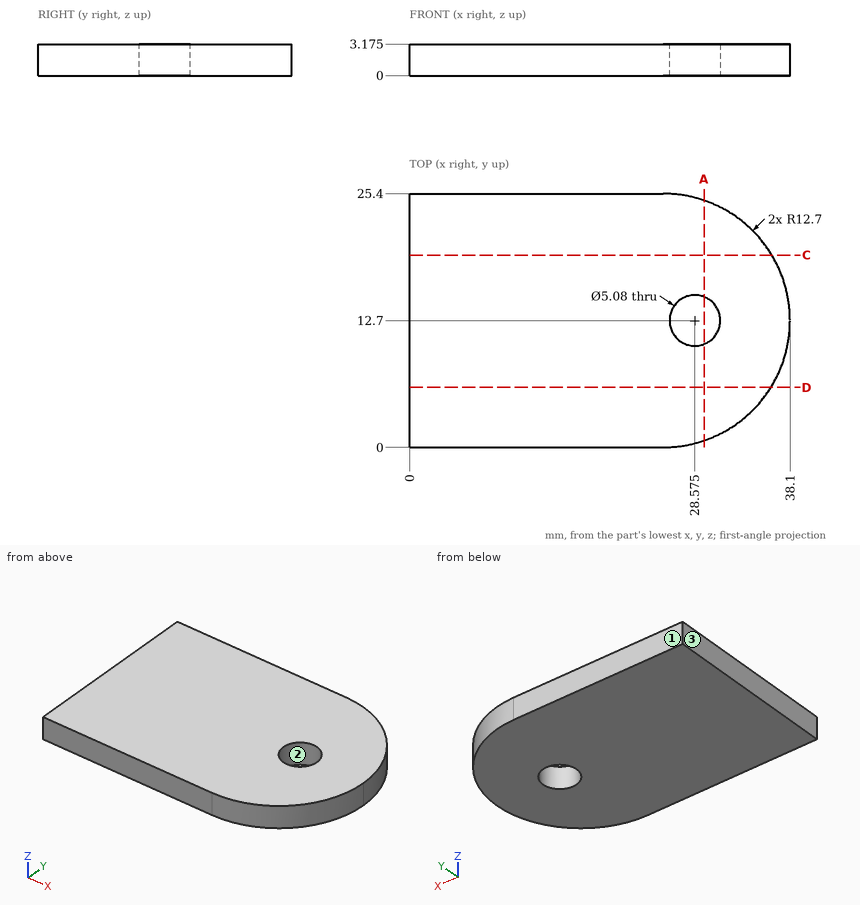
Input: dimensioned drawing with shaded views. Units: mm. Origin: part minimum x, y, z. Coordinates: 2 decimals unless noted, no trailing zeros. Loops run counter-clockwise (first coordinate to the right, second up) from the corner with the lowest first, then second, coordinate; pieces in that order, holes last. Notation, with made-up numbers: M 13.25,-35.5 L 50.25,-35.5 A23 cw 50.25,-24.5 Z; hole C 78.25,-12.75 d6. An arc over 180 degrees is marked long. Use a Markdown table: item, result. Add a question column.
Q1. Draft query along X for the marked faces 1, 2 and 3. Return one class per face: pulls with the +X half, pulls with the -X half, needs draft (parallel to the pull), parting line crosses it, or undercut.
Q2. Section query C-C, the plane y = 19.25. Return loops of the section in (x, z) (1 decimal), and give its area (3 significant figures).
Q3. Section query D-D, the plane y = 6. Return loops of the section in (x, z) (3 decimals), and give its area (3 significant figures).
Q4. Material intervals for L1, parallel to X at y = 12.5, z = 2.4; L2, parallel to X at y = 12, z = 2.55; L3, parallel to X at y = 9.5, z = 2.45, sorted ascending.
Q5. Section query A-A, the plane x = 29.5. Return loops of the section in (y, z) (1 decimal), and give its area (3 significant figures).
Result:
| question | item | result |
|---|---|---|
| 1 | face 1 | needs draft |
| 1 | face 2 | undercut |
| 1 | face 3 | pulls with the -X half |
| 2 | outline | M 0,0 L 36.3,0 L 36.3,3.2 L 0,3.2 Z |
| 2 | area | 115 mm2 |
| 3 | outline | M 0,0 L 36.189,0 L 36.189,3.175 L 0,3.175 Z |
| 3 | area | 115 mm2 |
| 4 | L1 | x = 0 to 26.04, 31.11 to 38.1 |
| 4 | L2 | x = 0 to 26.13, 31.02 to 38.08 |
| 4 | L3 | x = 0 to 37.69 |
| 5 | outline | M 0.7,0 L 10.3,0 L 10.3,3.2 L 0.7,3.2 Z; M 15.1,0 L 24.7,0 L 24.7,3.2 L 15.1,3.2 Z |
| 5 | area | 61.3 mm2 |
